from build123d import *

# Parameters (mm, degrees)
SKETCH1_W           = 23.2
SKETCH1_H           = 5.8
BOSS_EXTRUDE1_DEPTH = 13
SKETCH2_R           = 7.5
SKETCH2_W           = 18
SKETCH2_H           = 5.61118816
CUT_EXTRUDE1_DEPTH  = 19.36300629
SKETCH3_W           = 20.6
SKETCH3_H           = 4.4
CUT_EXTRUDE2_DEPTH  = 11
SKETCH4_W           = 0.8
SKETCH4_H           = 0.2
BOSS_EXTRUDE2_DEPTH = 3
FILLET1_R           = 1
SKETCH5_W           = 5
SKETCH5_H           = 15.702848837
BOSS_EXTRUDE3_DEPTH = 0.2
SKETCH6_W           = 5
SKETCH6_H           = 0.2
BOSS_EXTRUDE4_DEPTH = 3
FILLET2_R           = 0.5


with BuildPart() as part:
    # Sketch1 → Boss-Extrude1 (new body)
    with BuildSketch(Plane(origin=(0, 0, 0), x_dir=(1, 0, 0), z_dir=(0, 1, 0))):
        Rectangle(SKETCH1_W, SKETCH1_H)
    extrude(amount=BOSS_EXTRUDE1_DEPTH)

    # Sketch2 → Cut-Extrude1 (cut, through all)
    with BuildSketch(Plane.XY.offset(2.9)):
        with Locations((0, 13)):
            Circle(SKETCH2_R)
        with Locations((0, -1.80559408)):
            Rectangle(SKETCH2_W, SKETCH2_H)
    extrude(amount=-CUT_EXTRUDE1_DEPTH, mode=Mode.SUBTRACT)

    # Sketch3 → Cut-Extrude2 (cut)
    with BuildSketch(Plane(origin=(0, 13, 0), x_dir=(1, 0, 0), z_dir=(0, 1, 0))):
        Rectangle(SKETCH3_W, SKETCH3_H)
    extrude(amount=-CUT_EXTRUDE2_DEPTH, mode=Mode.SUBTRACT)

    # Sketch4 → Boss-Extrude2 (add)
    with BuildSketch(Plane.XZ.offset(-1)):
        with Locations((0, 1.27)):
            Rectangle(SKETCH4_W, SKETCH4_H)
        with Locations((-5.08, -1.27)):
            Rectangle(SKETCH4_W, SKETCH4_H)
        with Locations((5.08, -1.27)):
            Rectangle(SKETCH4_W, SKETCH4_H)
    extrude(amount=BOSS_EXTRUDE2_DEPTH)

    # Fillet1
    fillet1_edges = [part.edges().sort_by_distance(p)[0] for p in [
        (11.6, 6.5, 2.9),
        (-11.6, 6.5, 2.9),
        (-11.6, 6.5, -2.9),
        (11.6, 6.5, -2.9),
    ]]
    fillet(fillet1_edges, radius=FILLET1_R)

    # Sketch5 → Boss-Extrude3 (add)
    with BuildSketch(Plane.XY.offset(-2.2)):
        with Locations((-7.8, 13.148575582)):
            Rectangle(SKETCH5_W, SKETCH5_H)
    extrude(amount=BOSS_EXTRUDE3_DEPTH)

    # Sketch6 → Boss-Extrude4 (add)
    with BuildSketch(Plane.XY.offset(-2)):
        with Locations((-7.8, 20.9)):
            Rectangle(SKETCH6_W, SKETCH6_H)
    extrude(amount=BOSS_EXTRUDE4_DEPTH)

    # Fillet2
    fillet2_edges = [part.edges().sort_by_distance(p)[0] for p in [
        (-7.8, 21, -2.2),
    ]]
    fillet(fillet2_edges, radius=FILLET2_R)


solid = part.part
Can you work these out from the model? Positions are in its coordinate system, mm. A direction names the side the tool comes from. Coordinates: 2 decimals unless noted, no trailing zeros. Order: outer loops, then holes, each group sorted by start corner. A loop starts at its lowest first (then second) coordinate and runs counter-clockwise, first axis right, second up. Notation, with made-up numbers: M 34.25,54.25 L 75.25,54.25 A25 cw 75.25,88.25 Z; hole C 6,85.5 d10. An arc over 180 degrees is marked long. Write item = value, one per line.
(1) Suppose I cut it at C-C on y = 9.5. Please give me the cut outline in (x, z).
Results are:
outline = M -11.6,-1.9 A1 ccw -10.6,-2.9 L -6.63,-2.9 L -6.63,-2.2 L -5.3,-2.2 L -5.3,-2 L -10.3,-2 L -10.3,2.2 L -6.63,2.2 L -6.63,2.9 L -10.6,2.9 A1 ccw -11.6,1.9 Z; M 6.63,-2.9 L 10.6,-2.9 A1 ccw 11.6,-1.9 L 11.6,1.9 A1 ccw 10.6,2.9 L 6.63,2.9 L 6.63,2.2 L 10.3,2.2 L 10.3,-2.2 L 6.63,-2.2 Z
(2) I need wall thicknesses on line 1 along X through (y, z) = (12.25, 0); line 2 along Z through (x, y) = (10, 5); line 3 along Y through (x, z) = (0.5, 0.4). Which ranges of each line are inside material? Lowest first, please. Write a range as [from, to].
Results are:
line_1 = [-11.6, -10.3], [10.3, 11.6]
line_2 = [-2.9, -2.2], [2.2, 2.9]
line_3 = [1, 2]
(3) Suppose I cut it at D-D on x = 0. Please give me the cut outline in (y, z), plus the area to 3 significant figures.
Results are:
outline = M -2,1.17 L 1,1.17 L 1,-2.9 L 5.5,-2.9 L 5.5,-2.2 L 2,-2.2 L 2,2.2 L 5.5,2.2 L 5.5,2.9 L 1,2.9 L 1,1.37 L -2,1.37 Z
area = 11.3 mm2
(4) For pin 1 Ø2.5 at (y, z) = (17, -1) entering from +X; pin 2 Ø2 at (x, z) = (2.5, 0.5) entering from -Y; pin 3 Ø1.3 at (x, z) = (9.5, 0) entering from -Y, each with a flat end and sliding along its axis, tell me the tip position at first contact or that it passes through.
Results are:
pin_1 = -5.3
pin_2 = 1
pin_3 = 0
(5) Suppose I cut it at A-A on y = 3.5. Please give me the cut outline in (x, z).
Results are:
outline = M -11.6,-1.9 A1 ccw -10.6,-2.9 L 10.6,-2.9 A1 ccw 11.6,-1.9 L 11.6,1.9 A1 ccw 10.6,2.9 L -10.6,2.9 A1 ccw -11.6,1.9 Z; hole M -10.3,-2.2 L 10.3,-2.2 L 10.3,2.2 L -10.3,2.2 Z
(6) For faces 1 (the face through (-5, 0, -1.37)), 2 (the face through (5, 0, -1.17)), 3 (the face through (-8, 20.8, -1)), which set-ups out of +Z, -Z, +X, -X, +Y, -Y let a thin tool reach every point of the face, with its end or its side?
Results are:
face_1 = -Z, -Y
face_2 = +Z, -Y
face_3 = +Z, +X, -X
(7) Suppose I cut it at B-B on z = -0.75. Please give me the cut outline in (x, y), plus the area to 3 significant figures.
Results are:
outline = M -11.6,0 L -9,0 L -9,1 L 9,1 L 9,0 L 11.6,0 L 11.6,13 L 10.3,13 L 10.3,2 L -10.3,2 L -10.3,13 L -11.6,13 Z; M -10.3,20.8 L -5.3,20.8 L -5.3,21 L -10.3,21 Z
area = 58.0 mm2
(8) If we mould it in two halves opening along Z, with no side actions, what happens to faces 4 (the face through (0, 2, 0)), 5 (the face through (9, 0.5, 0)), 6 (the face through (5, 0, -1.37))? For each: pulls with the +Z half, pulls with the -Z half, needs draft (parallel to the pull), parting line crosses it, or undercut.
Results are:
face_4 = undercut
face_5 = needs draft
face_6 = pulls with the -Z half
